from build123d import *

# Parameters (mm, degrees)
ESBO_O1_W                        = 93
ESBO_O1_H                        = 88
RESSALTO_EXTRUS_O2_DEPTH         = 35
ESBO_O1_5_W                      = 93
ESBO_O1_5_H                      = 88
RESSALTO_EXTRUS_O3_DEPTH         = 8
ESBO_O1_7_R                      = 2
RESSALTO_EXTRUS_O6_DEPTH         = 8
ESBO_O4_R                        = 2.218632056
RESSALTO_EXTRUS_O7_DEPTH         = 4
ESBO_O5_W                        = 88.65
ESBO_O5_H                        = 82.92
RESSALTO_EXTRUS_O8_DEPTH         = 2
ESBO_O7_W                        = 12.6
ESBO_O7_H                        = 15.81
CORTE_EXTRUS_O1_DEPTH            = 154.290573748
ESBO_O8_W                        = 12.6
ESBO_O8_H                        = 15.81
CORTE_EXTRUS_O2_DEPTH            = 154.290573748
FURO_COM_FOLGA_DE_41_D           = 3.2639
FURO_COM_FOLGA_DE_41_DEPTH       = 8
FURO_COM_FOLGA_DE_41_CSINK_D     = 4.5339
FURO_COM_FOLGA_DE_41_CSINK_ANGLE = 90
FURO_COM_FOLGA_DE_41_TIP         = 0.980574487


with BuildPart() as part:
    # Esbo_o1 → Ressalto-extrus_o2 (new body)
    with BuildSketch(Plane(origin=(0, 0, 0), x_dir=(1, 0, 0), z_dir=(0, 1, 0))):
        with BuildLine():
            Line((0, -3), (93, -3))
            ThreePointArc((93, -3), (95.121320344, -2.121320344), (96, 0))
            Line((96, 0), (96, 88))
            ThreePointArc((96, 88), (95.121320344, 90.121320344), (93, 91))
            Line((93, 91), (0, 91))
            ThreePointArc((0, 91), (-2.121320344, 90.121320344), (-3, 88))
            Line((-3, 88), (-3, 0))
            ThreePointArc((-3, 0), (-2.121320344, -2.121320344), (0, -3))
        make_face()
        with Locations((46.5, 44)):
            Rectangle(ESBO_O1_W, ESBO_O1_H, mode=Mode.SUBTRACT)
    extrude(amount=RESSALTO_EXTRUS_O2_DEPTH)

    # Esbo_o1_5 → Ressalto-extrus_o3 (add)
    with BuildSketch(Plane(origin=(0, 0, 0), x_dir=(1, 0, 0), z_dir=(0, 1, 0))):
        with Locations((46.5, 44)):
            Rectangle(ESBO_O1_5_W, ESBO_O1_5_H)
    extrude(amount=RESSALTO_EXTRUS_O3_DEPTH)

    # Esbo_o1_7 → Ressalto-extrus_o6 (add)
    # profile 1 of 2: a face of its own
    with BuildSketch(Plane(origin=(0, 0, 0), x_dir=(1, 0, 0), z_dir=(0, 1, 0))):
        with BuildLine():
            Line((-13, 38.5), (-3, 38.5))
            Line((-3, 38.5), (-3, 49.5))
            Line((-3, 49.5), (-13, 49.5))
            ThreePointArc((-13, 49.5), (-14.414213562, 48.914213562), (-15, 47.5))
            Line((-15, 47.5), (-15, 40.5))
            ThreePointArc((-15, 40.5), (-14.414213562, 39.085786438), (-13, 38.5))
        make_face()
        with Locations(Location((-8.5, 44, 0), (0, 0, 270))):
            Circle(ESBO_O1_7_R, mode=Mode.SUBTRACT)
    # profile 2 of 2: a face of its own
    with BuildSketch(Plane(origin=(0, 0, 0), x_dir=(1, 0, 0), z_dir=(0, 1, 0))):
        with BuildLine():
            Line((96, 49.5), (96, 38.5))
            Line((96, 38.5), (106, 38.5))
            ThreePointArc((106, 38.5), (107.414213562, 39.085786438), (108, 40.5))
            Line((108, 40.5), (108, 47.5))
            ThreePointArc((108, 47.5), (107.414213562, 48.914213562), (106, 49.5))
            Line((106, 49.5), (96, 49.5))
        make_face()
        with Locations(Location((101.5, 44, 0), (0, 0, 270))):
            Circle(ESBO_O1_7_R, mode=Mode.SUBTRACT)
    extrude(amount=RESSALTO_EXTRUS_O6_DEPTH)

    # Esbo_o4 → Ressalto-extrus_o7 (add)
    # profile 1 of 2: a face of its own
    with BuildSketch(Plane(origin=(0, 35, 0), x_dir=(1, 0, 0), z_dir=(0, 1, 0))):
        with BuildLine():
            Line((41, -3), (52, -3))
            Line((52, -3), (52, -13))
            ThreePointArc((52, -13), (51.414213562, -14.414213562), (50, -15))
            Line((50, -15), (43, -15))
            ThreePointArc((43, -15), (41.585786438, -14.414213562), (41, -13))
            Line((41, -13), (41, -3))
        make_face()
        with Locations(Location((46.5, -8.5, 0), (0, 0, 270))):
            Circle(ESBO_O4_R, mode=Mode.SUBTRACT)
    # profile 2 of 2: a face of its own
    with BuildSketch(Plane(origin=(0, 35, 0), x_dir=(1, 0, 0), z_dir=(0, 1, 0))):
        with BuildLine():
            Line((43, 103), (50, 103))
            ThreePointArc((50, 103), (51.414213562, 102.414213562), (52, 101))
            Line((52, 101), (52, 91))
            Line((52, 91), (41, 91))
            Line((41, 91), (41, 101))
            ThreePointArc((41, 101), (41.585786438, 102.414213562), (43, 103))
        make_face()
        with Locations(Location((46.5, 96.5, 0), (0, 0, 90))):
            Circle(ESBO_O4_R, mode=Mode.SUBTRACT)
    extrude(amount=-RESSALTO_EXTRUS_O7_DEPTH)

    # Esbo_o5 → Ressalto-extrus_o8 (add)
    with BuildSketch(Plane(origin=(0, 8, 0), x_dir=(1, 0, 0), z_dir=(0, 1, 0))):
        with Locations((46.5, 44)):
            Rectangle(ESBO_O5_W, ESBO_O5_H)
    extrude(amount=RESSALTO_EXTRUS_O8_DEPTH)

    # Esbo_o7 → Corte-extrus_o1 (cut, through all)
    with BuildSketch(Plane.XY.offset(-88)):
        with Locations((67.38, 15.905)):
            Rectangle(ESBO_O7_W, ESBO_O7_H)
        with Locations((84.02, 15.905)):
            Rectangle(ESBO_O7_W, ESBO_O7_H)
    extrude(amount=-CORTE_EXTRUS_O1_DEPTH, mode=Mode.SUBTRACT)

    # Esbo_o8 → Corte-extrus_o2 (cut, through all)
    with BuildSketch(Plane(origin=(0, 0, 0), x_dir=(-1, 0, 0), z_dir=(0, 0, -1))):
        with Locations((-76.29, 15.905)):
            Rectangle(ESBO_O8_W, ESBO_O8_H)
    extrude(amount=-CORTE_EXTRUS_O2_DEPTH, mode=Mode.SUBTRACT)

    # Furo com folga de _41
    with Locations(Plane(origin=(6.12, 10, -82.28), x_dir=(0, 0, 1), z_dir=(0, 1, 0))):
        with Locations((0, 0), (76.45, 0), (76.45, 80.77)):
            CounterSinkHole(FURO_COM_FOLGA_DE_41_D / 2, FURO_COM_FOLGA_DE_41_CSINK_D / 2, depth=FURO_COM_FOLGA_DE_41_DEPTH, counter_sink_angle=FURO_COM_FOLGA_DE_41_CSINK_ANGLE)
            with Locations((0, 0, -(FURO_COM_FOLGA_DE_41_DEPTH + FURO_COM_FOLGA_DE_41_TIP / 2))):  # 118° drill point
                Cone(0, FURO_COM_FOLGA_DE_41_D / 2, FURO_COM_FOLGA_DE_41_TIP, mode=Mode.SUBTRACT)


solid = part.part
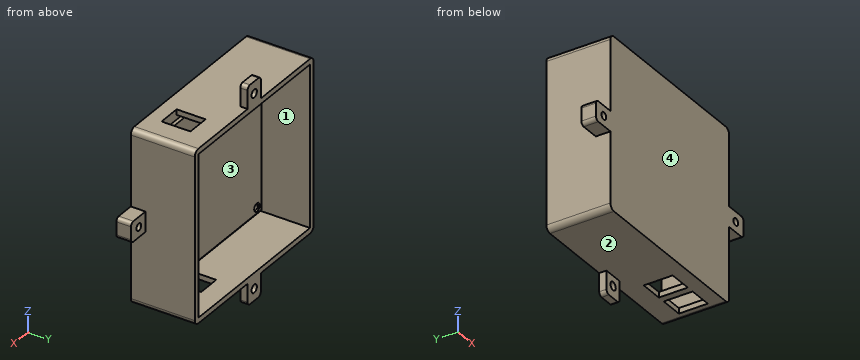
Geometry: final body of the model. Coordinates: model frame, mm. Face numbers are marked on the shaded views. A direction names the side the tool comes from. Round coordinates to 2 decimals unless told otherwise and drop trailing zeros. Loops run counter-clockwise (first coordinate to the right, second up) from the corner with the lowest first, then second, coordinate; pieces in that order, holes last. Notation, with made-up numbers: (11, 86.25) -> (36, 86.25) arc R21 ccw to (36, 113.25) -> close; hole circle Ø6 at (48.5, -5.5). An arc over 180 degrees is marked (long way). One line per question, with ' | ' between items. Start each with the question number.
1. Section D-D on y = 20. Output: boundary loops of the cut face in (x, z), and give its area (3 significant figures).
2. Section A-A on x = 46.5. Output: boundary loops of the cut face in (y, z).
3. Contact query for flat-ended pins moving along their axis: pin 1 (1.2 mm diameter, centred on y = 32.5, z = 9, fed in from +X); pin 2 (0.9 mm diameter, centred on y = 13.5, z = -89.5, fed in from -X); pin 3 (4 mm diameter, centred on y = 19, z = -38.5, fed in from +X). Output: stop coordinate, or through.
4. Mould query, pull axis X, two halves, no side actions, for the marked faces 1 and 2. Classes: pulls with the +X half, pulls with the -X half, needs draft (parallel to the pull), parting line crosses it, or undercut.
5. Section C-C on z = -96.5. Output: boundary loops of the cut face in (x, y).
6. Section B-B on y = 28. Output: boundary loops of the cut face in (x, z).
7. Line query: line 1 along Z through (x, y) = (6, 5); line 2 along Z through (x, y) = (54, 10.5); line 3 along X through (y, z) = (5, -82). Output: solid intervals per line, ascending. Write a range as [from, to].
8. Set-up query: the marked faces 3 and 4. Return all of +Z, -Z, +X, -X, +Y, -Y with unobstructed straight access to the full face (end or side cutting, diameter ignored); none if empty.
Returned:
1) outline: (-3, -88) arc R3 ccw to (0, -91) -> (61.08, -91) -> (61.08, -88) -> (0, -88) -> (0, 0) -> (69.99, 0) -> (69.99, 3) -> (0, 3) arc R3 ccw to (-3, 0) -> close; (73.68, -91) -> (77.72, -91) -> (77.72, -88) -> (73.68, -88) -> close; (82.59, 0) -> (93, 0) -> (93, -88) -> (90.32, -88) -> (90.32, -91) -> (93, -91) arc R3 ccw to (96, -88) -> (96, 0) arc R3 ccw to (93, 3) -> (82.59, 3) -> close | area: 1,000 mm2
2) outline: (0, -91) -> (31, -91) -> (31, -94.28) -> (35, -94.28) -> (35, -88) -> (8, -88) -> (8, -85.46) -> (10, -85.46) -> (10, -2.54) -> (8, -2.54) -> (8, 0) -> (35, 0) -> (35, 6.28) -> (31, 6.28) -> (31, 3) -> (0, 3) -> close; (31, -103) -> (35, -103) -> (35, -98.72) -> (31, -98.72) -> close; (31, 10.72) -> (35, 10.72) -> (35, 15) -> (31, 15) -> close
3) pin 1: stops at x = 52 | pin 2: stops at x = -2.81 | pin 3: stops at x = 96
4) face 1: undercut | face 2: needs draft
5) outline: (41, 31) -> (44.28, 31) -> (44.28, 35) -> (41, 35) -> close; (48.72, 31) -> (52, 31) -> (52, 35) -> (48.72, 35) -> close
6) outline: (-3, -88) arc R3 ccw to (0, -91) -> (93, -91) arc R3 ccw to (96, -88) -> (96, 0) arc R3 ccw to (93, 3) -> (0, 3) arc R3 ccw to (-3, 0) -> close; hole (0, -88) -> (93, -88) -> (93, 0) -> (0, 0) -> close
7) line 1: z = [-91, -83.91], [-80.65, -7.46], [-4.2, 3] | line 2: z = [-91, -88], [0, 3] | line 3: x = [-3, 4.51], [7.73, 96]
8) face 3: +Y | face 4: +Z, -Z, +X, -X, -Y
